from build123d import *

# Parameters (mm, degrees)
F0_R     = 6
F1_DEPTH = 2
F2_SIZE2 = 2.5980762114
F2_SIZE  = 1.5
F4_R     = 2.35
F4_R_2   = 1.4
F5_DEPTH = 4.5
F6_R     = 1.2


# Not quite as in the source:
# - a fillet or chamfer that OpenCascade refuses, or shapes differently, is made with other operations: its cross-section is extruded or revolved along the edge and cut away or added


with BuildPart() as f1:
    # F0 (on Top) → F1 (new body)
    with BuildSketch(Plane.XY):
        Circle(F0_R)
    extrude(amount=F1_DEPTH)

    # F2
    f2_edges = [f1.edges().sort_by_distance(p)[0] for p in [
        (-6, 0, 0),
    ]]
    f2_side = f1.faces().sort_by_distance((-6, 0, 1))[0]
    chamfer(f2_edges, length=F2_SIZE, length2=F2_SIZE2, reference=f2_side)

    # F3: fillet of radius 1 on 2 edges, made by hand

    # F3_s1 → F3_t2 (revolve, cut)
    with BuildSketch(Plane.XZ):
        with BuildLine():
            ThreePointArc((3.6339745962, 0.1339745962), (3.3927936413, 0.0340741737), (3.1339745962, 0))
            Line((3.1339745962, 0), (3.4019237886, 0))
            Line((3.4019237886, 0), (3.6339745962, 0.1339745962))
        make_face()
    revolve(axis=Axis((0, 0, 0), (0, 0, 1)), mode=Mode.SUBTRACT)

    # F3_s3 → F3_t4 (revolve, cut)
    with BuildSketch(Plane.XZ):
        with BuildLine():
            ThreePointArc((6, 2), (5.8486778537, 1.5452494356), (5.5031382462, 1.2131367327))
            Line((5.5031382462, 1.2131367327), (6, 1.5))
            Line((6, 1.5), (6, 2))
        make_face()
    revolve(axis=Axis((0, 0, 1.5), (0, 0, 1)), mode=Mode.SUBTRACT)

    # F4 (on face) → F5 (join)
    with BuildSketch(Plane.XY.offset(2)):
        Circle(F4_R)
        Circle(F4_R_2, mode=Mode.SUBTRACT)
    extrude(amount=F5_DEPTH)

    # F6
    f6_edges = [f1.edges().sort_by_distance(p)[0] for p in [
        (-1.4, 0, 2),
    ]]
    fillet(f6_edges, radius=F6_R)


solid = f1.part
The listing builds one solid part. Answer for the finished solid, in the listing's coordinates (mm). A direction names the side the tool comes from. Give positions to 0.01 mm unless a question says otherwise; leave off trailing zeros. Write each loop counter-clockwise with the first axis right and the second up, starting at its lowest first coordinate (ties: lowest second). Pieces come first, ordered by that corner, then holes. Notation, with made-up numbers: (28, 68.5) - (84, 68.5) arc R15 ccw to (84, 74.5) - close; hole circle Ø6 at (61.25, -38.75). An arc over 180 degrees is marked (long way). Use a Markdown table: item, result.
1. Section B-B on z = 1.5 is taken. Write down the section's boundary in (x, y).
Values follow:
| item | result |
|---|---|
| outline | circle Ø11.64 at (0, 0) |
2. A tool of negligible diameter and unlimited length cuts with its end or side. For faces 1 (the flat face through (0, -2, 6.5)), 2 (the flat face through (3, 0, 2)), from which of +Z, -Z, +X, -X, +Y, -Y can it reach the whole face along a straight path? Write none if from no direction.
Values follow:
| item | result |
|---|---|
| face 1 | +Z, +X, -X, +Y, -Y |
| face 2 | +Z |
3. Section A-A on z = 5 is taken. Write down the section's boundary in (x, y), plus the area to 3 significant figures.
Values follow:
| item | result |
|---|---|
| outline | circle Ø4.7 at (0, 0); hole circle Ø2.8 at (0, 0) |
| area | 11.2 mm² |
4. Each of these flat-tipped pins is pushed along its axis until it touches: P1, Ø1.5, axis at y = 4.5, z = 1.5, coming from the -X side; P2, Ø3, axis at x = 4, y = -0.5, coming from the +Z side. Where does it stop, or does it pass through?
Values follow:
| item | result |
|---|---|
| P1 | stops at x = -4.59 |
| P2 | stops at z = 2 |
5. For a pull along Y with two mould halves and no side action, classify faces 3 (the cylindrical face through (-0.509, -2.294, 4.219)), 4 (the cylindrical face through (-1.4, 0.06, 4.83)), 5 (the flat face through (0, 0, 0)) as released by +Y, released by -Y, zero draft, split by the parting line, or undercut.
Values follow:
| item | result |
|---|---|
| face 3 | split by the parting line |
| face 4 | undercut |
| face 5 | zero draft |
6. Find the intervals of material crossed by probe 1 along Y at (x, z) = (0, 4.75); probe 2 along X at (y, z) = (0.5, 3); probe 3 along X at (y, z) = (0.25, 5.25), in increasing order. Write a range as from..to.
Values follow:
| item | result |
|---|---|
| probe 1 | y = -2.35..-1.4, 1.4..2.35 |
| probe 2 | x = -2.3..-1.29, 1.29..2.3 |
| probe 3 | x = -2.34..-1.38, 1.38..2.34 |
